```python
from build123d import *

# Parameters (mm, degrees)
ESQUISSE1_R        = 177
BOSS_EXTRU_1_DEPTH = 89
ESQUISSE2_R        = 5.5
BOSS_EXTRU_2_DEPTH = 200
BOSS_EXTRU_4_DEPTH = 1


with BuildPart() as part:
    # Esquisse1 → Boss.-Extru.1 (new body)
    with BuildSketch(Plane.XY):
        Circle(ESQUISSE1_R)
    extrude(amount=BOSS_EXTRU_1_DEPTH)

    # Esquisse2 → Boss.-Extru.2 (add)
    with BuildSketch(Plane.XY.offset(89)):
        with Locations((-131.939733982, -3.988307506)):
            Circle(ESQUISSE2_R)
        with Locations((78.648083604, -106.011692494)):
            Circle(ESQUISSE2_R)
        with Locations((131.939733982, 3.988307506)):
            Circle(ESQUISSE2_R)
        with Locations((-78.648083604, 106.011692494)):
            Circle(ESQUISSE2_R)
    extrude(amount=BOSS_EXTRU_2_DEPTH)

    # Esquisse4 → Boss.-Extru.4 (add)
    with BuildSketch(Plane.XY.offset(89)):
        Polygon((-29.640529762, 82.269024992), (-29.858528448, 81.819051023), (15.138868472, 60.019182436), (15.356867158, 60.469156405), align=None)
    extrude(amount=BOSS_EXTRU_4_DEPTH)


solid = part.part
```
Geometry check sheet. Reference: the model listing, model coordinates, mm. A direction names the side the tool comes from. Give positions to 0.01 mm unless a question says otherwise; leave off trailing zeros. Write each loop counter-clockwise with the first axis right and the second up, starting at its lowest first coordinate (ties: lowest second). Pieces come first, ordered by that corner, then holes. Notation, with made-up numbers: (10.5, -2.75) -> (30.5, -2.75) arc R27 cw to (30.5, 18.25) -> close; hole circle Ø5 at (47.5, -25). An arc over 180 degrees is marked (long way). Use one line per item in the form item = value.
Item 1: Sectioned sample at B-B on z = 103. Enter the section's corners in (x, y).
Results list:
outline = circle Ø11 at (-131.94, -3.99); circle Ø11 at (-78.65, 106.01); circle Ø11 at (78.65, -106.01); circle Ø11 at (131.94, 3.99)
Item 2: Mould release check, pull along X, two halves, no side actions. Record for faces 4 (the flat face through (-6.83, 71.22, 89.49)), 5 (the cylindrical face through (137.2, 5.6, 187.6)), 6 (the flat face through (-2, 2, 0)), 7 (the cylindrical face through (-38.37, -172.79, 43.88)): released by +X, released by -X, zero draft, split by the parting line, or undercut.
Results list:
face_4 = released by +X
face_5 = undercut
face_6 = zero draft
face_7 = split by the parting line
Item 3: Sectioned sample at C-C on y = -124.5. Enter the section's corners in (x, z), plus the area to 3 significant figures.
Results list:
outline = (-125.81, 0) -> (125.81, 0) -> (125.81, 89) -> (-125.81, 89) -> close
area = 22,400 mm2
Item 4: Sectioned sample at D-D on x = 47. Enter the section's corners in (y, z), plus the area to 3 significant figures.
Results list:
outline = (-170.65, 0) -> (170.65, 0) -> (170.65, 89) -> (-170.65, 89) -> close
area = 30,400 mm2
Item 5: Scan lines: line 1 (Z direction, x = 59.5, y = -105.5); line 2 (Y direction, x = -131, z = 112); line 3 (Y direction, x = 135, z = 48.5). Record each from-to range of solid material in increasing order.
Results list:
line_1 = 0 to 89
line_2 = -9.41 to 1.43
line_3 = -114.47 to 114.47
Item 6: Access from +Z, -Z, +X, -X, +Y, -Y to the whole of each face (thin tool, end or side, straight path). Record for faces 1 (the cylindrical face through (-82.7, 109.73, 187.6)), 2 (the flat face through (-132, -4, 289)), 3 (the flat face through (-7.67, 71.07, 89.49)).
Results list:
face_1 = +Z
face_2 = +Z, +X, -X, +Y, -Y
face_3 = +Z, -X, -Y
Item 7: Depth check by flat-ended pin: pin 1 Ø5 at (x, z) = (139.5, 243.5) entering from -Y; pin 2 Ø6.5 at (x, y) = (-4.5, 66) entering from +Z; pin 3 Ø5 at (x, z) = (-84.5, 111.5) entering from +Y. Enter the tip coordinate at first touch or a pass-through.
Results list:
pin_1 = 1.83
pin_2 = 90
pin_3 = 110.37
Item 8: Sectioned sample at A-A on x = -12. Enter the section's corners in (y, z), plus the area to 3 significant figures.
Results list:
outline = (-176.59, 0) -> (176.59, 0) -> (176.59, 89) -> (73.72, 89) -> (73.72, 90) -> (73.17, 90) -> (73.17, 89) -> (-176.59, 89) -> close
area = 31,400 mm2
